Geometry check sheet. Reference: the model listing, model coordinates, mm. Give positions to 0.01 mm unless a question says otherwise; leave off trailing zeros. Write each loop counter-clockwise with the first axis right and the second up, starting at its lowest first coordinate (ties: lowest second). Pieces come first, ordered by that corner, then holes. Notation, with made-up numbers: (-19.75, 55) - (25.25, 55) arc R28 ccw to (25.25, 94) - close; hole circle Ø5 at (32, 63.25). An arc over 180 degrees is marked (long way). Use a Markdown table: item, result.
Autodesk Inventor part; units mm, degrees
ref_plane "YZ Plane" through (0, 0, 0) normal (1, 0, 0) x (0, 1, 0)
ref_plane "XZ Plane" through (0, 0, 0) normal (0, 1, 0) x (-1, 0, 0)
ref_plane "XY Plane" through (0, 0, 0) normal (0, 0, 1) x (1, 0, 0)
sketch "Sketch1: base" plane through (0, 0, 0) normal (0, 0, 1) x (1, 0, 0)
  line L0 (-22.9459, 27.4044) -> (22.0541, 27.4044)
  line L1 (22.0541, 27.4044) -> (22.0541, -17.5956)
  line L2 (22.0541, -17.5956) -> (-22.9459, -17.5956)
  line L3 (-22.9459, -17.5956) -> (-22.9459, 27.4044)
  circle A0 centre (-0.4459, 4.9044) radius 16.375
  line L4 (-16.4459, 20.9044) -> (15.5541, 20.9044) construction
  line L5 (15.5541, 20.9044) -> (15.5541, -11.0956) construction
  line L6 (15.5541, -11.0956) -> (-16.4459, -11.0956) construction
  line L7 (-16.4459, -11.0956) -> (-16.4459, 20.9044) construction
  circle A1 centre (-0.4459, 4.9044) radius 14.875
  circle A2 centre (15.5541, 20.9044) radius 1.8 construction
  circle A3 centre (15.5541, 20.9044) radius 3.25 construction
  point P0 (0, 0)
  point P1 (22.0541, 4.9044)
  point P2 (-0.4459, 27.4044)
  point P3 (-0.4459, 20.9044)
  point P4 (-16.4459, 4.9044)
  dimension "d0" = 32.75
  dimension "d1" = 45
  dimension "d4" = 32
  dimension "d16" = 1.5
  dimension "d19" = 6.5
  dimension "d20" = 3.6
  dimension "d21" = 6.5
extrude "Ex1: base" add sketch "Sketch1: base" along normal blind 5 contours L0 L1 L2 L3
hole "Hole1: M3 screws" at (-16.4459, 20.9044, 0) at (15.5541, 20.9044, 0) at (-16.4459, -11.0956, 0) at (15.5541, -11.0956, 0) direction (0, 0, 1) diameter 3.6 end through all counterbore diameter 6.5 counterbore depth 3
fillet "Fillet1" radius 2 8 edges at (-0.4459, 27.4044, 0) (22.0541, 4.9044, 0) (22.0541, 27.4044, 2.5) (-22.9459, 4.9044, 0) (-0.4459, -17.5956, 0) (22.0541, -17.5956, 2.5) (-22.9459, -17.5956, 2.5) (-22.9459, 27.4044, 2.5)
extrude "Ex2: stopper" add sketch "Sketch1: base" along normal blind 0.8 contours A0
fillet "Fillet2 (for printing)" radius 0.8 1 edges at (-16.8209, 4.9044, 0.8)
properties part number "cage_inside_01"
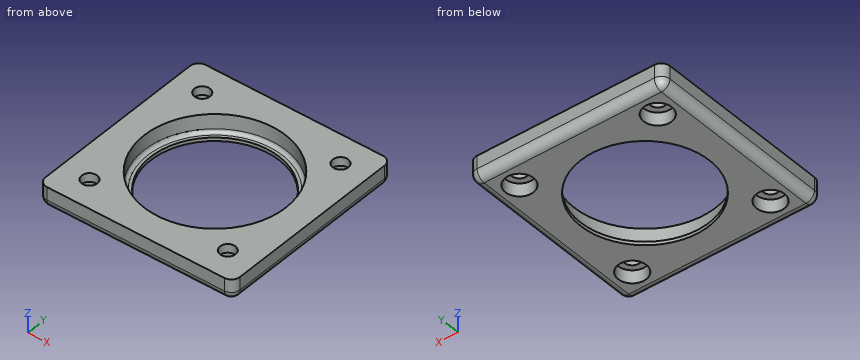
1) Material ranges on L1, parallel to Y at x = -13.5, z = 1.9; L2, parallel to Y at x = 14, z = 1.8; L3, parallel to X at y = 14, z = 4.45, recorded low to high. Write a range as from..to.
Working result:
| item | result |
|---|---|
| L1 | y = -17.59..-12.47, -9.72..-4.98, 14.79..19.53, 22.28..27.4 |
| L2 | y = -17.59..-13.95, -8.24..-2.81, 12.62..18.05, 23.76..27.39 |
| L3 | x = -22.95..-14.06, 13.17..22.05 |
2) Section check A-A on z = 3.85. Record the boundary of the cut face in (x, y) (3 decimals), then the cut area to 3 significant figures.
Working result:
| item | result |
|---|---|
| outline | (-22.946, -15.596) arc R2 ccw to (-20.946, -17.596) - (20.054, -17.596) arc R2 ccw to (22.054, -15.596) - (22.054, 25.404) arc R2 ccw to (20.054, 27.404) - (-20.946, 27.404) arc R2 ccw to (-22.946, 25.404) - close; hole circle Ø3.6 at (-16.446, -11.096); hole circle Ø3.6 at (-16.446, 20.904); hole circle Ø32.75 at (-0.446, 4.904); hole circle Ø3.6 at (15.554, -11.096); hole circle Ø3.6 at (15.554, 20.904) |
| area | 1,140 mm² |
3) Section check B-B on x = -17.5. Record the boundary of the cut face in (y, z).
Working result:
| item | result |
|---|---|
| outline | (-17.6, 2) arc R2 ccw to (-15.6, 0) - (-14.17, 0) - (-14.17, 3) - (-12.55, 3) - (-12.55, 5) - (-17.6, 5) - close; (-9.64, 3) - (-8.02, 3) - (-8.02, 0) - (17.83, 0) - (17.83, 3) - (19.45, 3) - (19.45, 5) - (-9.64, 5) - close; (22.36, 3) - (23.98, 3) - (23.98, 0) - (25.4, 0) arc R2 ccw to (27.4, 2) - (27.4, 5) - (22.36, 5) - close |
4) Section check D-D on y = 23.5. Record the boundary of the cut face in (x, z).
Working result:
| item | result |
|---|---|
| outline | (-22.95, 2) arc R2 ccw to (-20.95, 0) - (-18.4, 0) - (-18.4, 3) - (-14.49, 3) - (-14.49, 0) - (13.6, 0) - (13.6, 3) - (17.51, 3) - (17.51, 0) - (20.05, 0) arc R2 ccw to (22.05, 2) - (22.05, 5) - (-22.95, 5) - close |
5) Section check C-C on y = -13.5. Record the boundary of the cut face in (x, z).
Working result:
| item | result |
|---|---|
| outline | (-22.95, 2) arc R2 ccw to (-20.95, 0) - (-18.63, 0) - (-18.63, 3) - (-14.26, 3) - (-14.26, 0) - (13.37, 0) - (13.37, 3) - (17.74, 3) - (17.74, 0) - (20.05, 0) arc R2 ccw to (22.05, 2) - (22.05, 5) - (-22.95, 5) - close |
6) Depth check by flat-ended pin: P1, Ø5, axis at x = 15, y = -11.5, coming from the -Z side; P2, Ø3, axis at x = 15.55, y = -11.1, coming from the -Z side; P3, Ø8, axis at x = -7, y = -5, coming from the +Z side. Enter the tip coordinate at first touch or a pass-through.
Working result:
| item | result |
|---|---|
| P1 | stops at z = 3 |
| P2 | passes through |
| P3 | stops at z = 0.86 |
